```python
from build123d import *

# Parameters (mm, degrees)
F0_W     = 114.3
F0_H     = 76.2
F1_DEPTH = 38.1
F2_R     = 38.1
F3_SIZE  = 12.7
F4_W     = 32.1010919288
F4_H     = 12.0379095897
F5_DEPTH = 90.932


with BuildPart() as f1:
    # F0 (on Front) → F1 (new body, symmetric)
    with BuildSketch(Plane.XZ):
        with Locations((-0.4010554403, -6.0710595265)):
            Rectangle(F0_W, F0_H)
    extrude(amount=F1_DEPTH, both=True)

    # F2
    f2_edges = [f1.edges().sort_by_distance(p)[0] for p in [
        (-0.401055, -38.1, 32.02894),
    ]]
    fillet(f2_edges, radius=F2_R)

    # F3
    f3_edges = [f1.edges().sort_by_distance(p)[0] for p in [
        (56.748945, 19.05, 32.02894),
    ]]
    chamfer(f3_edges, length=F3_SIZE)

    # F4 (on Front) → F5 (join)
    with BuildSketch(Plane.XZ):
        with Locations((-4.5737079345, 16.7265743949)):
            Rectangle(F4_W, F4_H)
    extrude(amount=F5_DEPTH)


solid = f1.part
```
Input: part model. Units: mm. Frame: model coordinates. A direction names the side the tool comes from. Give positions to 0.01 mm unless a question says otherwise; leave off trailing zeros. Order: outer loops, then holes, each group sorted by start corner. A loop starts at its lowest first (then second) coordinate and runs counter-clockwise, first axis right, second up. Notation, with made-up numbers: M 55,66 L 72,66 A5 ccw 72,72 Z; hole C -2,76 d9. An arc over 180 degrees is marked long. One line per question, with ' | ' between items. Start each with the question number.
1. First-contact query: pin 1 Ø10 at (x, y) = (12, -40.5) entering from +Z; pin 2 Ø13 at (y, z) = (-67.5, 18) entering from +X; pin 3 Ø4 at (x, z) = (40, -25) entering from -Y; pin 4 Ø10 at (y, z) = (-41, -32.5) entering from -X. Flat tips, straight axial feed; report the tip coordinate or a pass-through.
2. Section query A-A (x = -17). Return the cut outline in (y, z), and give its area (3 significant figures).
3. Material intervals for probe 1 along Y at (x, z) = (-44.5, -18.5); probe 2 along X at (y, z) = (-37.5, 11); probe 3 along Z at (x, y) = (-17, -66.5), sorted ascending. Write a range as [from, to].
4. Pull-direction query (Z, two-part tool) for faces 4 (the face through (-1, 38.1, -6)), 5 (the face through (50.49, 18.78, 25.59)), 6 (the face through (-1, -1, -44.171)), 7 (the face through (-6.04, -22.195, 24.896)); classes: released by +Z, released by -Z, zero draft, split by the parting line, or undercut.
5. Section query B-B (z = -36.5). Return the cut outline in (x, y), and give its area (3 significant figures).
6. Section query D-D (x = 23). Return the cut outline in (y, z), and give its area (3 significant figures).
7. Section query C-C (y = -67.5). Return the cut outline in (x, z), and give its area (3 significant figures).
8. Access query for faces 1 (the face through (-7, -38.1, -25)), 2 (the face through (-20.624, -57, 17)), 3 (the face through (-5, -57, 22.746)). Directions: +Z, -Z, +X, -X, +Y, -Y. A direction counts if a zero-diameter tool reaches every point of the face in a straight line with its end or side. Return the directions, or none.
Here are the results:
1) pin 1: z = 22.75 | pin 2: x = 11.48 | pin 3: y = -38.1 | pin 4: x = -57.55
2) outline: M -90.93,10.71 L -34.21,10.71 A38.1 ccw -38.1,-6.07 L -38.1,-44.17 L 38.1,-44.17 L 38.1,32.03 L 0,32.03 A38.1 ccw -24.92,22.75 L -90.93,22.75 Z | area: 6,230 mm²
3) probe 1: [-38.1, 38.1] | probe 2: [-20.62, 11.48] | probe 3: [10.71, 22.75]
4) face 4: zero draft | face 5: released by +Z | face 6: released by -Z | face 7: undercut
5) outline: M -57.55,-38.1 L 44.05,-38.1 L 56.75,-25.4 L 56.75,38.1 L -57.55,38.1 Z | area: 8,630 mm²
6) outline: M -38.1,-44.17 L 38.1,-44.17 L 38.1,32.03 L 0,32.03 A38.1 ccw -38.1,-6.07 Z | area: 5,490 mm²
7) outline: M -20.62,10.71 L 11.48,10.71 L 11.48,22.75 L -20.62,22.75 Z | area: 386 mm²
8) face 1: -Z, +X, -X, -Y | face 2: +Z, -X, -Y | face 3: +Z, +X, -X, -Y
